from build123d import *

# Parameters (mm, degrees)
SKETCH1_W           = 40
SKETCH1_H           = 40
BOSS_EXTRUDE1_DEPTH = 3
SKETCH2_R           = 5.875
BOSS_EXTRUDE2_DEPTH = 5
SKETCH3_W           = 3.5
SKETCH3_H           = 19
BOSS_EXTRUDE3_DEPTH = 20
SKETCH4_R           = 3
CUT_EXTRUDE1_DEPTH  = 3.5
FILLET1_R           = 2.5
CHAMFER1_SIZE       = 2.5


with BuildPart() as part:
    # Sketch1 → Boss-Extrude1 (new body)
    with BuildSketch(Plane(origin=(0, 0, 0), x_dir=(1, 0, 0), z_dir=(0, 1, 0))):
        Rectangle(SKETCH1_W, SKETCH1_H)
    extrude(amount=BOSS_EXTRUDE1_DEPTH)

    # Sketch2 → Boss-Extrude2 (add)
    with BuildSketch(Plane(origin=(0, 3, 0), x_dir=(1, 0, 0), z_dir=(0, 1, 0))):
        Circle(SKETCH2_R)
    extrude(amount=BOSS_EXTRUDE2_DEPTH)

    # Sketch3 → Boss-Extrude3 (add)
    with BuildSketch(Plane(origin=(0, 3, 0), x_dir=(1, 0, 0), z_dir=(0, 1, 0))):
        with Locations((15.15, 0)):
            Rectangle(SKETCH3_W, SKETCH3_H)
    boss_extrude3 = extrude(amount=BOSS_EXTRUDE3_DEPTH)

    # Sketch4 → Cut-Extrude1 (cut)
    with BuildSketch(Plane(origin=(16.9, 0, 0), x_dir=(0, 0, -1), z_dir=(1, 0, 0))):
        with Locations((0, 18)):
            Circle(SKETCH4_R)
    cut_extrude1 = extrude(amount=-CUT_EXTRUDE1_DEPTH, mode=Mode.SUBTRACT)

    # Fillet1
    fillet1_edges = [part.edges().sort_by_distance(p)[0] for p in [
        (20, 1.5, 20),
        (-20, 1.5, 20),
        (-20, 1.5, -20),
        (20, 1.5, -20),
    ]]
    fillet(fillet1_edges, radius=FILLET1_R)

    # Mirror1: Boss-Extrude3, Cut-Extrude1 across plane
    add(boss_extrude3.mirror(Plane(origin=(0, 0, 0), x_dir=(0, 0, 1), z_dir=(1, 0, 0))))
    add(cut_extrude1.mirror(Plane(origin=(0, 0, 0), x_dir=(0, 0, 1), z_dir=(1, 0, 0))), mode=Mode.SUBTRACT)

    # Chamfer1
    chamfer1_edges = [part.edges().sort_by_distance(p)[0] for p in [
        (15.15, 23, -9.5),
        (15.15, 23, 9.5),
        (-15.15, 23, 9.5),
        (-15.15, 23, -9.5),
    ]]
    chamfer(chamfer1_edges, length=CHAMFER1_SIZE)


solid = part.part
Model file for the job. Use its own axes, mm. A direction names the side the tool comes from. Coordinates: 2 decimals unless noted, no trailing zeros. Order: outer loops, then holes, each group sorted by start corner. A loop starts at its lowest first (then second) coordinate and runs counter-clockwise, first axis right, second up. Notation, with made-up numbers: (74.25, -10) -> (111.25, -10) arc R20 ccw to (111.25, 9) -> close; hole circle Ø7 at (52, -6.5). An arc over 180 degrees is marked (long way). Return JSON: item names as keys, results as strings. Group by question number.
Item 1: Wall check: line 1 along X through (y, z) = (14.5, -8); line 2 along Y through (x, z) = (15.5, 16.5); line 3 along Y through (x, z) = (-16, 0). Give the ranges that are in metal, low to high. Write a range as [from, to].
Item 2: Saw through at A-A on z = 0. Write the cut outline in (x, y) (3 decimals), then the cut area to 3 significant figures.
Item 3: Saw through at C-C on y = 18. Write the cut outline in (x, z), then the cut area to 3 significant figures.
Item 4: Saw through at D-D on y = 6.25. Write the cut outline in (x, z) (3 decimals), then the cut area to 3 significant figures.
Item 5: Flat gauge pins, fed straight in: P1, Ø3.5, axis at x = 2, z = 0, coming from the +Y side; P2, Ø4, axis at x = 15, y = 14, coming from the +Z side; P3, Ø1, axis at x = -10, z = 0, coming from the +Y side. Where does each tip first touch, or does it go through?
Item 6: Pull direction Z, two halves, no side cores. Call faces 5 (the flat face through (-15, 23, 0)), 6 (the cylindrical face through (15.17, 15.07, 0.65)), 7 (the flat face through (-15, 22, 8)): pulls with the +Z half, pulls with the -Z half, needs draft (parallel to the pull), parting line crosses it, or undercut.
Item 7: Saw through at B-B on x = -16. Write the cut outline in (y, z), then the cut area to 3 significant figures.
Item 8: Tool access for faces 1 (the flat face through (-15, 12, -9.5)), 2 (the cylindrical face through (5.604, 5.465, -1.765)), 3 (the flat face through (15, 12, 9.5)), 4 (the flat face through (16.9, 13, 0)): list every direction of +Z, -Z, +X, -X, +Y, -Y with a clear straight run to the whole face (end or side of a thin tool).
Values found:
{
 "1": {"line 1": "x = [-16.9, -13.4], [13.4, 16.9]", "line 2": "y = [0, 3]", "line 3": "y = [0, 15], [21, 23]"},
 "2": {"outline": "(-20, 0) -> (20, 0) -> (20, 3) -> (16.9, 3) -> (16.9, 15) -> (13.4, 15) -> (13.4, 3) -> (5.875, 3) -> (5.875, 8) -> (-5.875, 8) -> (-5.875, 3) -> (-13.4, 3) -> (-13.4, 15) -> (-16.9, 15) -> (-16.9, 3) -> (-20, 3) -> close; (-16.9, 21) -> (-13.4, 21) -> (-13.4, 23) -> (-16.9, 23) -> close; (13.4, 21) -> (16.9, 21) -> (16.9, 23) -> (13.4, 23) -> close", "area": "277 mm2"},
 "3": {"outline": "(-16.9, -9.5) -> (-13.4, -9.5) -> (-13.4, -3) -> (-16.9, -3) -> close; (-16.9, 3) -> (-13.4, 3) -> (-13.4, 9.5) -> (-16.9, 9.5) -> close; (13.4, -9.5) -> (16.9, -9.5) -> (16.9, -3) -> (13.4, -3) -> close; (13.4, 3) -> (16.9, 3) -> (16.9, 9.5) -> (13.4, 9.5) -> close", "area": "91.0 mm2"},
 "4": {"outline": "(-16.9, -9.5) -> (-13.4, -9.5) -> (-13.4, 9.5) -> (-16.9, 9.5) -> close; circle Ø11.75 at (0, 0); (13.4, -9.5) -> (16.9, -9.5) -> (16.9, 9.5) -> (13.4, 9.5) -> close", "area": "241 mm2"},
 "5": {"P1": "stops at y = 8", "P2": "stops at z = 9.5", "P3": "stops at y = 3"},
 "6": {"face 5": "needs draft", "face 6": "undercut", "face 7": "pulls with the +Z half"},
 "7": {"outline": "(0, -20) -> (3, -20) -> (3, -9.5) -> (20.5, -9.5) -> (23, -7) -> (23, 7) -> (20.5, 9.5) -> (3, 9.5) -> (3, 20) -> (0, 20) -> close; hole circle Ø6 at (18, 0)", "area": "465 mm2"},
 "8": {"face 1": "-Z, +X, -X, +Y", "face 2": "+Y", "face 3": "+Z, +X, -X, +Y", "face 4": "+Z, -Z, +X, +Y"}
}
